```python
from build123d import *

# Parameters (mm, degrees)
F0_W     = 30
F0_H     = 16.5
F0_R     = 2
F1_DEPTH = 1
F2_DEPTH = 3.5
F3_W     = 30
F3_H     = 1.75
F4_DEPTH = 2.5
F5_R     = 8


with BuildPart() as f1:
    # F0 (on Top) → F1 (new body)
    with BuildSketch(Plane.XY):
        Rectangle(F0_W, F0_H)
        with Locations((-12.5, 0)):
            Circle(F0_R, mode=Mode.SUBTRACT)
        with Locations((12.5, 0)):
            Circle(F0_R, mode=Mode.SUBTRACT)
        with Locations((-12.5, 0)):
            Circle(F0_R)
        with Locations((12.5, 0)):
            Circle(F0_R)
    extrude(amount=F1_DEPTH)

    # F0 (on Top) → F2 (join)
    with BuildSketch(Plane.XY):
        with Locations((-12.5, 0)):
            Circle(F0_R)
        with Locations((12.5, 0)):
            Circle(F0_R)
    extrude(amount=F2_DEPTH)

    # F3 (on face) → F4 (join)
    with BuildSketch(Plane.XY.offset(1)):
        with Locations((0, 7.375)):
            Rectangle(F3_W, F3_H)
        with Locations((0, -7.375)):
            Rectangle(F3_W, F3_H)
    extrude(amount=F4_DEPTH)

    # F5
    f5_edges = [f1.edges().sort_by_distance(p)[0] for p in [
        (-15, -8.25, 1.75),
        (-15, 8.25, 1.75),
        (15, -8.25, 1.75),
        (15, 8.25, 1.75),
    ]]
    fillet(f5_edges, radius=F5_R)


solid = f1.part
```
Work out the finished part from the listing and answer in its coordinate system (mm). A direction names the side the tool comes from. Round coordinates to 2 decimals unless told otherwise and drop trailing zeros. Loops run counter-clockwise (first coordinate to the right, second up) from the corner with the lowest first, then second, coordinate; pieces in that order, holes last. Notation, with made-up numbers: M 86,26 L 109,26 A38 cw 109,64 Z; hole C -17,14 d11. An arc over 180 degrees is marked long. Use CSV: the item, a comma, the result in double quotes.
Q1. Section B-B, the plane z = 0.7 is taken. Determine the outline of the cut face in (x, y), then the cut area to 3 significant figures.
Determined:
outline,"M -15,-0.25 A8 ccw -7,-8.25 L 7,-8.25 A8 ccw 15,-0.25 L 15,0.25 A8 ccw 7,8.25 L -7,8.25 A8 ccw -15,0.25 Z"
area,"440 mm2"
Q2. A tool of negligible diameter and unlimited length cuts with its end or side. For faces 1 (the flat face through (0, 0, 1)), 2 (the flat face through (0, -7, 3.5)), 3 (the flat face through (0, 6.5, 2)), from which of +Z, -Z, +X, -X, +Y, -Y can it reach the whole face along a straight path? Write none if from no direction.
Determined:
face 1,"+Z"
face 2,"+Z, +X, -X, +Y, -Y"
face 3,"+Z, +X, -X"
Q3. Section C-C, the plane x = -12.5 is taken. Determine the outline of the cut face in (y, z).
Determined:
outline,"M -6.06,0 L 6.06,0 L 6.06,1 L 2,1 L 2,3.5 L -2,3.5 L -2,1 L -6.06,1 Z"
Q4. Each of these flat-tipped pins is pushed along its axis until it touches: pin 1 (1 mm diameter, centred on x = 3, y = -1, fed in from +Z); pin 2 (2 mm diameter, centred on x = -10, z = 1.5, fed in from +Y). Where does it stop, or does it pass through?
Determined:
pin 1,"z = 1"
pin 2,"y = 8"
Q5. Section D-D, the plane y = 1 is taken. Determine the outline of the cut face in (x, z), then the cut area to 4 significant figures.
Determined:
outline,"M -14.96,0 L 14.96,0 L 14.96,1 L 14.23,1 L 14.23,3.5 L 10.77,3.5 L 10.77,1 L -10.77,1 L -10.77,3.5 L -14.23,3.5 L -14.23,1 L -14.96,1 Z"
area,"47.25 mm2"
Q6. Consider L1, parallel to Y at x = -5, z = 1.1; L2, parallel to Y at x = 10, z = 2.5; L3, parallel to Z at x = -8.5, y = -4.5. Determine where each line is inside the solid, lowest interval first.
Determined:
L1,"-8.25 to -6.5, 6.5 to 8.25"
L2,"-7.67 to -6.5, 6.5 to 7.67"
L3,"0 to 1"
Q7. The mould has two halves that part along X. Classify faces 4 (the cylindrical face through (-11.66, 6.752, 1.337)), 5 (the cylindrical face through (10.9, -1.2, 2.2)), 6 (the cylindrical face through (11.66, -6.752, 1.337)), 7 (the cylindrical face through (-14.1, -1.2, 2.2)): pulls with the +X half, pulls with the -X half, needs draft (parallel to the pull), parting line crosses it, or undercut.
Determined:
face 4,"pulls with the -X half"
face 5,"undercut"
face 6,"pulls with the +X half"
face 7,"undercut"
Q8. Section A-A, the plane z = 3.1 is taken. Determine the outline of the cut face in (x, y), then the cut area to 3 significant figures.
Determined:
outline,"C -12.5,0 d4; M -11.99,-6.5 A8 ccw -7,-8.25 L 7,-8.25 A8 ccw 11.99,-6.5 Z; M -11.99,6.5 L 11.99,6.5 A8 ccw 7,8.25 L -7,8.25 A8 ccw Z; C 12.5,0 d4"
area,"98.0 mm2"
